Model file for the job. Use its own axes, mm. A direction names the side the tool comes from. Give positions to 0.01 mm unless a question says otherwise; leave off trailing zeros. Write each loop counter-clockwise with the first axis right and the second up, starting at its lowest first coordinate (ties: lowest second). Pieces come first, ordered by that corner, then holes. Notation, with made-up numbers: (16, -28) - (43, -28) arc R29 ccw to (43, 5) - close; hole circle Ø7 at (6, 82). An arc over 180 degrees is marked (long way). Use a Markdown table: item, result. Add a question column.
```python
from build123d import *

# Parameters (mm, degrees)
SKETCH1_W           = 12.7
SKETCH1_H           = 80
SKETCH1_R           = 1.5
BOSS_EXTRUDE1_DEPTH = 12.7


with BuildPart() as part:
    # Sketch1 → Boss-Extrude1 (new body)
    with BuildSketch(Plane(origin=(572.952355873, -103.733491168, -119.473981867), x_dir=(0, 0, 1), z_dir=(1, 0, 0))):
        with Locations((-165.577945174, 149.370143232)):
            Rectangle(SKETCH1_W, SKETCH1_H)
        with Locations(Location((-165.577945174, 169.370143232, 0), (0, 0, 270))):
            Circle(SKETCH1_R, mode=Mode.SUBTRACT)
        with Locations(Location((-165.577945174, 184.370143232, 0), (0, 0, 270))):
            Circle(SKETCH1_R, mode=Mode.SUBTRACT)
        with Locations(Location((-165.577945174, 114.370143232, 0), (0, 0, 270))):
            Circle(SKETCH1_R, mode=Mode.SUBTRACT)
        with Locations(Location((-165.577945174, 129.370143232, 0), (0, 0, 270))):
            Circle(SKETCH1_R, mode=Mode.SUBTRACT)
        with BuildLine():
            Line((-162.077945174, 157.77541555), (-162.077945174, 140.964870914))
            ThreePointArc((-162.077945174, 140.964870914), (-165.577945174, 137.464870914), (-169.077945174, 140.964870914))
            Line((-169.077945174, 140.964870914), (-169.077945174, 157.77541555))
            ThreePointArc((-169.077945174, 157.77541555), (-165.577945174, 161.27541555), (-162.077945174, 157.77541555))
        make_face(mode=Mode.SUBTRACT)
    extrude(amount=BOSS_EXTRUDE1_DEPTH)


solid = part.part
```
(1) Band-saw the part on D-D (y = -218.5). Write the cut outline in (x, z).
(2) Two-plate mould, pull along Z, no slides. Class faces 1 (the cylindrical face through (579.213, -233.299, -283.565)), 2 (the flat face through (579, -293.104, -285)), 3 (the flat face through (579, -253, -291.402)): +Z half, -Z half, draft (parallel to the pull), parting line (faces both ways), or undercut.
(3) Band-saw the part on A-A (y = -258). Write the cut outline in (x, z), then the cut area to 3 significant figures.
(4) Band-saw the part on B-B (z = -284.25). Write the cut outline in (x, y).
(5) Which spindle directions (+Z, -Z, +X, -X, +Y, -Y) get a long thin tool onto all of the face, cutting with end or side? Do faces 4 (the flat face through (579, -253, -288.552)), 5 (the flat face through (585.652, -254, -289)). Say none if no direction does.
(6) Probe probe 1 along Y at (x, z) = (580.5, -285); probe 2 along Y at (x, z) = (578.75, -284); probe 3 along Z at (x, y) = (581.75, -248.5). List the from-to ranges inside material, lowest first. Write a range as [from, to].
(7) Band-saw the part on C-C (x = 576). Write the cut outline in (y, z), then the cut area to 3 significant figures.
Model answer:
| question | item | result |
|---|---|---|
| 1 | outline | (572.95, -291.4) - (585.65, -291.4) - (585.65, -286.5) - (572.95, -286.5) - close; (572.95, -283.61) - (585.65, -283.61) - (585.65, -278.7) - (572.95, -278.7) - close |
| 2 | face 1 | undercut |
| 2 | face 2 | draft |
| 2 | face 3 | -Z half |
| 3 | outline | (572.95, -291.4) - (585.65, -291.4) - (585.65, -288.55) - (572.95, -288.55) - close; (572.95, -281.55) - (585.65, -281.55) - (585.65, -278.7) - (572.95, -278.7) - close |
| 3 | area | 72.4 mm^2 |
| 4 | outline | (572.95, -293.1) - (585.65, -293.1) - (585.65, -289.37) - (572.95, -289.37) - close; (572.95, -286.84) - (585.65, -286.84) - (585.65, -274.37) - (572.95, -274.37) - close; (572.95, -271.84) - (585.65, -271.84) - (585.65, -264.92) - (572.95, -264.92) - close; (572.95, -241.29) - (585.65, -241.29) - (585.65, -234.37) - (572.95, -234.37) - close; (572.95, -231.84) - (585.65, -231.84) - (585.65, -219.37) - (572.95, -219.37) - close; (572.95, -216.84) - (585.65, -216.84) - (585.65, -213.1) - (572.95, -213.1) - close |
| 5 | face 4 | +X, -X |
| 5 | face 5 | +Z, -Z, +X, +Y, -Y |
| 6 | probe 1 | y = [-293.1, -289.6], [-286.6, -274.6], [-271.6, -265.01], [-241.2, -234.6], [-231.6, -219.6], [-216.6, -213.1] |
| 6 | probe 2 | y = [-293.1, -289.17], [-287.03, -274.17], [-272.03, -264.85], [-241.36, -234.17], [-232.03, -219.17], [-217.03, -213.1] |
| 6 | probe 3 | z = [-291.4, -288.55], [-281.55, -278.7] |
| 7 | outline | (-293.1, -291.4) - (-213.1, -291.4) - (-213.1, -278.7) - (-293.1, -278.7) - close; hole circle Ø3 at (-288.1, -285.05); hole circle Ø3 at (-273.1, -285.05); hole (-261.51, -288.55) - (-244.7, -288.55) arc R3.5 ccw to (-244.7, -281.55) - (-261.51, -281.55) arc R3.5 ccw to start; hole circle Ø3 at (-233.1, -285.05); hole circle Ø3 at (-218.1, -285.05) |
| 7 | area | 832 mm^2 |
